Check sheet for the modelled part. Datum: model origin and axes. Units: mm. Face numbers are marked on the shaded views. Round coordinates to 2 decimals unless told otherwise and drop trailing zeros. Write each loop counter-clockwise with the first axis right and the second up, starting at its lowest first coordinate (ties: lowest second). Pieces come first, ordered by that corner, then holes. Notation, with made-up numbers: (8, 82.5) -> (20, 82.5) arc R26 cw to (20, 99.5) -> close; hole circle Ø11 at (-24.75, 62.5). An arc over 180 degrees is marked (long way). One line per item, written item: value.
from build123d import *

# Parameters (mm, degrees)
BOSS_EXTRUDE1_DEPTH = 10.5
BOSS_EXTRUDE3_START = 10.5
BOSS_EXTRUDE3_DEPTH = 10.5
SKETCH5_W           = 6
SKETCH5_H           = 6.5
CUT_EXTRUDE1_DEPTH  = 400
CUT_EXTRUDE2_DEPTH  = 40
CUT_EXTRUDE3_DEPTH  = 40


with BuildPart() as part:
    # Sketch2 → Boss-Extrude1 (new body)
    with BuildSketch(Plane(origin=(0, 0, 0), x_dir=(1, 0, 0), z_dir=(0, 1, 0))):
        with BuildLine():
            Line((-186.825, 51.625), (-186.825, -52.625))
            ThreePointArc((-186.825, -52.625), (-186.239213562, -54.039213562), (-184.825, -54.625))
            Line((-184.825, -54.625), (184.825, -54.625))
            ThreePointArc((184.825, -54.625), (186.239213562, -54.039213562), (186.825, -52.625))
            Line((186.825, -52.625), (186.825, 51.625))
            ThreePointArc((186.825, 51.625), (185.067640687, 55.867640687), (180.825, 57.625))
            Line((180.825, 57.625), (-180.825, 57.625))
            ThreePointArc((-180.825, 57.625), (-185.067640687, 55.867640687), (-186.825, 51.625))
        make_face()
        with BuildLine():
            ThreePointArc((-178.825, 47.625), (-179.532106781, 47.332106781), (-179.825, 46.625))
            Line((-179.825, 46.625), (-179.825, -46.625))
            ThreePointArc((-179.825, -46.625), (-179.532106781, -47.332106781), (-178.825, -47.625))
            Line((-178.825, -47.625), (178.825, -47.625))
            ThreePointArc((178.825, -47.625), (179.532106781, -47.332106781), (179.825, -46.625))
            Line((179.825, -46.625), (179.825, 46.625))
            ThreePointArc((179.825, 46.625), (179.532106781, 47.332106781), (178.825, 47.625))
            Line((178.825, 47.625), (-178.825, 47.625))
        make_face(mode=Mode.SUBTRACT)
    extrude(amount=BOSS_EXTRUDE1_DEPTH)

    # Sketch4 → Boss-Extrude3 (add)
    # profile 1 of 2: a face of its own
    with BuildSketch(Plane.XZ.offset(BOSS_EXTRUDE3_START)):
        with BuildLine():
            ThreePointArc((-184.825, 54.625), (-186.239213562, 54.039213562), (-186.825, 52.625))
            Line((-186.825, 52.625), (-186.825, -51.625))
            ThreePointArc((-186.825, -51.625), (-185.067640687, -55.867640687), (-180.825, -57.625))
            Line((-180.825, -57.625), (180.825, -57.625))
            ThreePointArc((180.825, -57.625), (185.067640687, -55.867640687), (186.825, -51.625))
            Line((186.825, -51.625), (186.825, 52.625))
            ThreePointArc((186.825, 52.625), (186.239213562, 54.039213562), (184.825, 54.625))
            Line((184.825, 54.625), (-184.825, 54.625))
        make_face()
        with BuildLine():
            Line((178.825, -47.625), (-178.825, -47.625))
            ThreePointArc((-178.825, -47.625), (-179.532106781, -47.332106781), (-179.825, -46.625))
            Line((-179.825, -46.625), (-179.825, 46.625))
            ThreePointArc((-179.825, 46.625), (-179.532106781, 47.332106781), (-178.825, 47.625))
            Line((-178.825, 47.625), (178.825, 47.625))
            ThreePointArc((178.825, 47.625), (179.532106781, 47.332106781), (179.825, 46.625))
            Line((179.825, 46.625), (179.825, -46.625))
            ThreePointArc((179.825, -46.625), (179.532106781, -47.332106781), (178.825, -47.625))
        make_face(mode=Mode.SUBTRACT)
    # profile 2 of 2: a face of its own
    with BuildSketch(Plane.XZ.offset(BOSS_EXTRUDE3_START)):
        with BuildLine():
            ThreePointArc((-178.825, -47.625), (-179.532106781, -47.332106781), (-179.825, -46.625))
            Line((-179.825, -46.625), (-179.825, 46.625))
            ThreePointArc((-179.825, 46.625), (-179.532106781, 47.332106781), (-178.825, 47.625))
            Line((-178.825, 47.625), (178.825, 47.625))
            ThreePointArc((178.825, 47.625), (179.532106781, 47.332106781), (179.825, 46.625))
            Line((179.825, 46.625), (179.825, -46.625))
            ThreePointArc((179.825, -46.625), (179.532106781, -47.332106781), (178.825, -47.625))
            Line((178.825, -47.625), (-178.825, -47.625))
        make_face()
    extrude(amount=-BOSS_EXTRUDE3_DEPTH)

    # Sketch5 → Cut-Extrude1 (cut)
    with BuildSketch(Plane(origin=(186.825, 0, 0), x_dir=(0, 0, -1), z_dir=(1, 0, 0))):
        Polygon((-52.625, -10.5), (-52.625, -0.219727509), (-54.625, 0), (-54.625, -10.5), align=None)
        Polygon((-52.625, -10.5), (40.947921748, -10.5), (-52.625, -0.219727509), align=None)
        Polygon((51.625, -10.5), (51.625, -4), (40.947921748, -10.5), align=None)
        with Locations((54.625, -7.25)):
            Rectangle(SKETCH5_W, SKETCH5_H)
    extrude(amount=-CUT_EXTRUDE1_DEPTH, mode=Mode.SUBTRACT)

    # Sketch6 → Cut-Extrude2 (cut)
    with BuildSketch(Plane(origin=(186.825, 0, 0), x_dir=(0, 0, -1), z_dir=(1, 0, 0))):
        Polygon((-54.625, 0), (51.625, -4), (40.947921748, -10.5), align=None)
    extrude(amount=-CUT_EXTRUDE2_DEPTH, mode=Mode.SUBTRACT)

    # Sketch7 → Cut-Extrude3 (cut)
    with BuildSketch(Plane.ZY.offset(186.825)):
        Polygon((-51.625, -4), (-40.947921748, -10.5), (52.625, -0.219727509), align=None)
    extrude(amount=-CUT_EXTRUDE3_DEPTH, mode=Mode.SUBTRACT)


solid = part.part
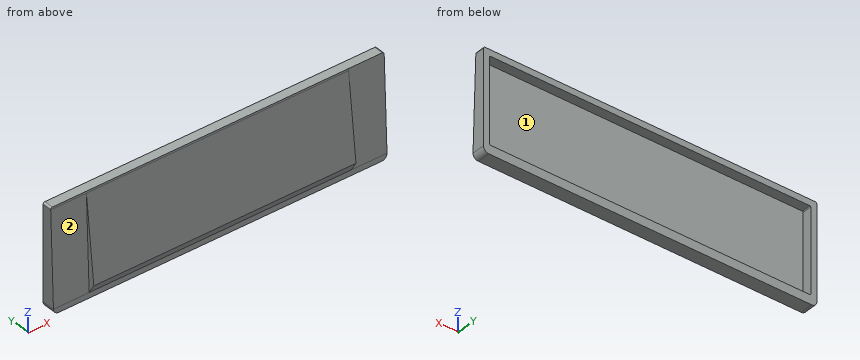
Item 1: Release check for a two-part mould opening along X. For the marked faces 1 and 2 record: pulls with the +X half, pulls with the -X half, needs draft (parallel to the pull), parting line crosses it, or undercut.
Result set:
face 1: undercut
face 2: needs draft
Item 2: Sectioned sample at C-C (z = -31). Enter the section's corners in (x, y) (3 decimals), then the cut area to 3 significant figures.
Result set:
outline: (-186.825, -3.252) -> (-146.825, -3.252) -> (-146.825, -9.407) -> (146.825, -9.407) -> (146.825, -3.224) -> (186.825, -3.224) -> (186.825, 10.5) -> (179.825, 10.5) -> (179.825, 0) -> (-179.825, 0) -> (-179.825, 10.5) -> (-186.825, 10.5) -> close
area: 3,170 mm^2
Item 3: Sectioned sample at A-A (x = 16.5). Enter the section's corners in (y, z) (3 decimals), then the cut area to 3 significant figures.
Result set:
outline: (-10.5, -40.948) -> (-4, -51.625) -> (-4, -57.625) -> (10.5, -57.625) -> (10.5, -47.625) -> (0, -47.625) -> (0, 47.625) -> (10.5, 47.625) -> (10.5, 54.625) -> (0, 54.625) -> close
area: 782 mm^2
Item 4: Material ranges on line 1 along X through (y, z) = (6.5, -23) (3 decimals); line 2 along Z through (x, y) = (116, 3.75) (3 decimals); line 3 along X through (y, z) = (-6, -39) (3 decimals), recorded low to high.
Result set:
line 1: -186.825 to -179.825, 179.825 to 186.825
line 2: -57.625 to -47.625, 47.625 to 54.625
line 3: -146.825 to 146.825
Item 5: Sectioned sample at B-B (z = 30). Enter the section's corners in (x, y) (3 decimals).
Result set:
outline: (-186.825, -1.04) -> (-146.825, -1.04) -> (-146.825, -2.705) -> (146.825, -2.705) -> (146.825, -0.927) -> (186.825, -0.927) -> (186.825, 10.5) -> (179.825, 10.5) -> (179.825, 0) -> (-179.825, 0) -> (-179.825, 10.5) -> (-186.825, 10.5) -> close
Item 6: Depth check by flat-ended pin: pin 1 (3 mm diameter, centred on x = 30, z = 22.5, fed in from -Y); pin 2 (12 mm diameter, centred on x = 27.5, z = -3, fed in from -Y); pin 3 (5 mm diameter, centred on x = -16.5, z = -54.5, fed in from -Y). Enter the tip coordinate at first touch or a pass-through.
Result set:
pin 1: y = -3.69
pin 2: y = -6.99
pin 3: y = -4
